```python
from build123d import *

# Parameters (mm, degrees)
F2_T = -2.5


with BuildPart() as f1:
    # F0 (on Front) → F1 (revolve)
    with BuildSketch(Plane.XZ):
        Polygon((-343.1598980381, -88.1673034342), (-343.1598980381, 11.8326965658), (-396.1598980381, 11.8326965658), (-396.1598980381, -91.1673034342), (-346.1598980381, -91.1673034342), (-346.1598980381, -88.1673034342), align=None)
    revolve(axis=Axis((-396.1598980381, 0, -39.6673034342), (0, 0, 1)))

    # F2
    f2_openings = [f1.faces().sort_by_distance(p)[0] for p in [
        (-396.159898, 0, 11.832697),
    ]]
    offset(amount=F2_T, openings=f2_openings, kind=Kind.INTERSECTION)


solid = f1.part
```
Check sheet for the modelled part. Datum: model origin and axes. Units: mm. A direction names the side the tool comes from. Give positions to 0.01 mm unless a question says otherwise; leave off trailing zeros. Order: outer loops, then holes, each group sorted by start corner. A loop starts at its lowest first (then second) coordinate and runs counter-clockwise, first axis right, second up. Notation, with made-up numbers: (4.25, 10) -> (25.25, 10) arc R22 cw to (25.25, 27) -> close; hole circle Ø4 at (39, 2.25). An arc over 180 degrees is marked (long way). Return JSON: item names as keys, results as strings.
1. Cross-section at C-C, the plane z = -74.5. Record the cut outline in (x, y).
From the geometry:
{"outline": "circle Ø106 at (-396.16, 0); hole circle Ø101 at (-396.16, 0)"}
2. Mould release check, pull along X, two halves, no side actions. Record for faces 1 (the cylindrical face through (-347.2, -20.3, -37.5)), 2 (the flat face through (-395, 1, -91.167)), 3 (the flat face through (-395, 1, -88.667)): +X half, -X half, draft (parallel to the pull), parting line (faces both ways), or undercut.
From the geometry:
{"face 1": "parting line", "face 2": "draft", "face 3": "undercut"}
3. Set-up check for faces 4 (the flat face through (-364.5, -39, -88.167)), 5 (the cylindrical face through (-443.614, 2.088, -87.146)), 6 (the flat face through (-349, -19, 11.833)): record each of +Z, -Z, +X, -X, +Y, -Y from which the full face is reachable in a straight line by a thin tool's end or side.
From the geometry:
{"face 4": "-Z", "face 5": "+Z", "face 6": "+Z, +X, -X, +Y, -Y"}
4. Material ranges on probe 1 along Z at (x, y) = (-430.5, -1); probe 2 along Y at (x, z) = (-388, -3); probe 3 along Y at (x, z) = (-407, -63), recorded low to high. Write a range as [from, to].
From the geometry:
{"probe 1": "[-91.17, -88.67]", "probe 2": "[-52.37, -49.84], [49.84, 52.37]", "probe 3": "[-51.88, -49.32], [49.32, 51.88]"}
5. Go/stop test with flat-tipped pins: P1, Ø4, axis at x = -365, z = -13, coming from the -Y side; P2, Ø8, axis at x = -356, y = 11.5, coming from the +Z side; P3, Ø5, axis at y = -3.5, z = -64, coming from the +X side. Record where each tip stops, or that it passes through.
From the geometry:
{"P1": "y = -44.26", "P2": "z = -88.67", "P3": "x = -343.17"}
6. Cross-section at B-B, the plane x = -406.5. Record the cut outline in (y, z).
From the geometry:
{"outline": "(-51.98, -88.17) -> (-48.92, -88.17) -> (-48.92, -91.17) -> (48.92, -91.17) -> (48.92, -88.17) -> (51.98, -88.17) -> (51.98, 11.83) -> (49.43, 11.83) -> (49.43, -85.67) -> (46.36, -85.67) -> (46.36, -88.67) -> (-46.36, -88.67) -> (-46.36, -85.67) -> (-49.43, -85.67) -> (-49.43, 11.83) -> (-51.98, 11.83) -> close"}
7. Cross-section at A-A, the plane y = 0. Record the cut outline in (x, z).
From the geometry:
{"outline": "(-449.16, -88.17) -> (-446.16, -88.17) -> (-446.16, -91.17) -> (-346.16, -91.17) -> (-346.16, -88.17) -> (-343.16, -88.17) -> (-343.16, 11.83) -> (-345.66, 11.83) -> (-345.66, -85.67) -> (-348.66, -85.67) -> (-348.66, -88.67) -> (-443.66, -88.67) -> (-443.66, -85.67) -> (-446.66, -85.67) -> (-446.66, 11.83) -> (-449.16, 11.83) -> close"}
